Build history of the part. All positions in model axes, mm. Face numbers are marked on the shaded views. A direction names the side the tool comes from. Round coordinates to 2 decimals unless told otherwise and drop trailing zeros. Write each loop counter-clockwise with the first axis right and the second up, starting at its lowest first coordinate (ties: lowest second). Pieces come first, ordered by that corner, then holes. Notation, with made-up numbers: M 28,25 L 66,25 A24 ccw 66,40 Z; hole C 21.5,40.25 d3. An arc over 180 degrees is marked long. One line per item, written item: value. Start each with the question number.
Autodesk Inventor part; units mm, degrees
ref_plane "YZ Plane" through (0, 0, 0) normal (1, 0, 0) x (0, 1, 0)
ref_plane "XZ Plane" through (0, 0, 0) normal (0, 1, 0) x (-1, 0, 0)
ref_plane "XY Plane" through (0, 0, 0) normal (0, 0, 1) x (1, 0, 0)
sketch "Sketch1" plane through (0, 0, 0) normal (0, 0, 1) x (1, 0, 0)
  circle A0 centre (9.5, 5) radius 0.75
  arc A1 (9.5, 1) -> (11.9441, 8.1664) centre (9.5, 5) ccw
  circle A2 centre (9.5, 5) radius 6.5 construction
  line L0 (9.5, 5) -> (-5.5, 5) construction
  circle A3 centre (-5.5, 5) radius 0.75
  line L1 (9.5, 1) -> (-9.5, 1)
  line L2 (-9.5, 1) -> (-9.5, 9)
  line L3 (-9.5, 9) -> (-9.5, 17)
  line L4 (-9.5, 17) -> (0.5, 17)
  line L5 (0.5, 17) -> (11.9441, 8.1664)
  point P0 (0, 0)
  dimension "d0" = 8
  dimension "d1" = 13
  dimension "d4" = 1.5
  dimension "d19" = 8
  dimension "d20" = 10
  dimension "d37" = 19
  dimension "d39" = 4
extrude "Extrusion1" add sketch "Sketch1" along normal blind 4
sketch "Sketch5" plane through (-9.5, 17, 0) normal (0, 1, 0) x (1, 0, 0)
  line L0 (10, 0) -> (0, 0)
  line L1 (0, 0) -> (0, -4)
  line L2 (10, -4) -> (0, -4)
  line L3 (10, 0) -> (10, -4)
  line L4 (0, 2) -> (10, 2)
  line L5 (10, 2) -> (10, -6)
  line L6 (10, -6) -> (0, -6)
  line L7 (0, -6) -> (0, 2)
  point P0 (9.5, 0)
  dimension "d40" = 2
  dimension "d41" = 8
  dimension "d42" = 10
extrude "Extrusion5" add sketch "Sketch5" against normal blind 16 contours L0 L7 L4 L5 | L5 L6 L7 L2
sketch "Sketch6" plane through (9.5, 1, 0) normal (0, -1, 0) x (1, 0, 0)
  line L0 (-9, 6) -> (-19, 6)
  line L1 (-19, 6) -> (-19, -2)
  line L2 (-19, -2) -> (-9, -2)
  line L3 (-9, -2) -> (-9, 0)
  line L4 (-19, 4) -> (-11, 4)
  line L5 (-11, 4) -> (-11, 0)
  line L6 (-11, 0) -> (-19, 0)
  point P0 (-9.5, 0)
  dimension "d45" = 2
  dimension "d46" = 2
  dimension "d47" = 8
extrude "Extrusion6" cut sketch "Sketch6" against normal blind 8
chamfer "Chamfer5" distance 2 angle 45 4 edges at (-9.5, 1, 5) (-9.5, 1, -1) (0.5, 17, 5) (0.5, 17, -1)
sketch "Sketch7" plane through (0.5, 17, 4) normal (0, 1, 0) x (1, 0, 0)
  line L0 (-10, 6) -> (-2, 6)
  line L1 (0, 4) -> (0, 0)
  circle A0 centre (-6, 2) radius 0.75
  point P0 (-8, 6)
  point P1 (-0.5, 4)
  dimension "d53" = 1.5
  dimension "d54" = 4
  dimension "d55" = 6
extrude "Extrusion7" cut sketch "Sketch7" against normal blind 6
sketch "Sketch8" plane through (-9.5, 17, 6) normal (0, 0, 1) x (1, 0, 0)
  line L0 (0, 0) -> (0, -14)
  line L1 (10, -16) -> (2, -16)
  circle A0 centre (4, -12) radius 0.75
  point P0 (9.5, -17)
  dimension "d58" = 1.5
  dimension "d59" = 4
  dimension "d60" = 4
extrude "Extrusion8" cut sketch "Sketch8" against normal blind 8
properties part number "Finger Joint"
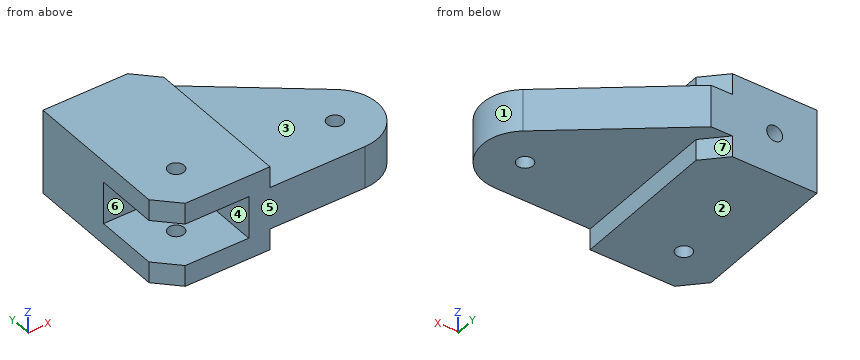
Item 1: Two-plate mould, pull along Z, no slides. Class the marked faces 1, 2, 3 and 4: pulls with the +Z half, pulls with the -Z half, needs draft (parallel to the pull), parting line crosses it, or undercut.
Item 2: Which spindle directions (+Z, -Z, +X, -X, +Y, -Y) get a long thin tool onto all of the face, cutting with end or side? Do the marked faces 5, 6 and 7. Say none if no direction does.
Item 3: Cut at D-D, the plane x = -0.5. Write the cut outline in (y, z).
Item 4: Cut at B-B, the plane z = 4.25. Write the cut outline in (x, y).
Item 5: Drill centre lines: line 1 (Z direction, x = -5.5, y = 12.25); line 2 (Z direction, x = -8.25, y = 3.5); line 3 (Z direction, x = 5.5, y = 8). Where is each one in solid material? Low to high.
Item 6: Cut at A-A, the plane y = 5. Write the cut outline in (x, z).
Item 7: Cut at C-C, the plane x = -5.5. Write the cut outline in (y, z), plus the area to 3 significant figures.
Item 8: Drop flat-ended pins along their axis: pin 1 (0.6 mm diameter, centred on y = 10, z = 5.5, fed in from +X); pin 2 (2.5 mm diameter, centred on x = 9.5, y = 5, fed in from -Z); pin 3 (1.2 mm diameter, centred on y = 4.5, z = 1, fed in from -X). Give the stop position or say it passes through.
Computed values:
1. face 1: needs draft
1. face 2: pulls with the -Z half
1. face 3: pulls with the +Z half
1. face 4: undercut
2. face 5: +Z, -Z, +X, -X, -Y
2. face 6: -X, -Y
2. face 7: -Z, +X, +Y
3. outline: M 1,-2 L 16,-2 L 16,0 L 17,0 L 17,4 L 16,4 L 16,6 L 1,6 Z
4. outline: M -9.5,3 L -7.5,1 L 0.5,1 L 0.5,15 L -1.5,17 L -9.5,17 Z; hole C -5.5,5 d1.5
5. line 1: z = -2 to 1.25, 2.75 to 6
5. line 2: z = -2 to 0, 4 to 6
5. line 3: z = 0 to 4
6. outline: M -9.5,-2 L -6.25,-2 L -6.25,0 L -9.5,0 Z; M -9.5,4 L -6.25,4 L -6.25,6 L -9.5,6 Z; M -4.75,-2 L 0.5,-2 L 0.5,0 L 8.75,0 L 8.75,4 L 0.5,4 L 0.5,6 L -4.75,6 L -4.75,4 L -1.5,4 L -1.5,0 L -4.75,0 Z; M 10.25,0 L 13.5,0 L 13.5,4 L 10.25,4 Z
7. outline: M 1,-2 L 4.25,-2 L 4.25,0 L 1,0 Z; M 1,4 L 4.25,4 L 4.25,6 L 1,6 Z; M 5.75,-2 L 17,-2 L 17,1.25 L 11,1.25 L 11,2.75 L 17,2.75 L 17,6 L 5.75,6 L 5.75,4 L 9,4 L 9,0 L 5.75,0 Z
7. area: 81.0 mm2
8. pin 1: stops at x = 0.5
8. pin 2: stops at z = 0
8. pin 3: stops at x = -1.5
